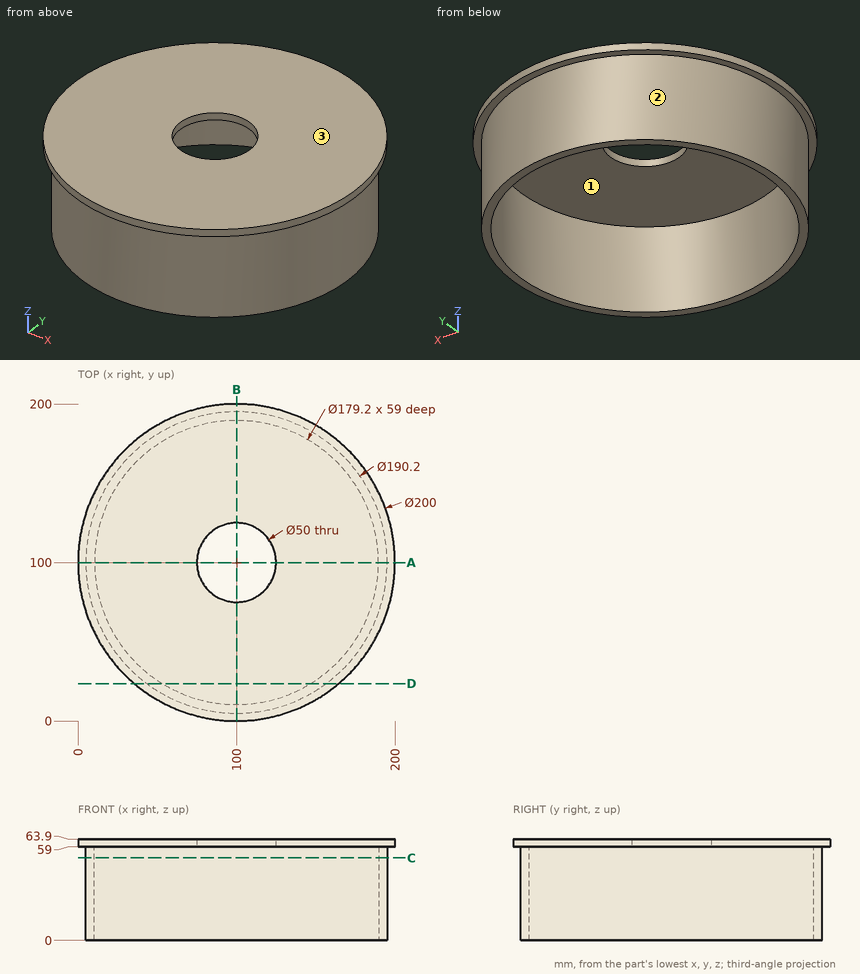
The figure shows three views and two pictorial views of one solid part (mm, origin at its lowest corner). Answer the questions. Give positions to 0.01 mm unless a question says otherwise; leave off trailing zeros. Loops run counter-clockwise (first coordinate to the right, second up) from the corner with the lowest first, then second, coordinate; pieces in that order, holes last. Notation, with made-up numbers: (-5, 73) -> (15, 73) arc R7 cw to (15, 83) -> close; hole circle Ø3 at (77, -6). An arc over 180 degrees is marked (long way). Use CSV: the item, a comma, the result in double quotes.
1. Straight lines are drawn through the part: line 1 (Y direction, x = 100, z = 62); line 2 (Y direction, x = 100, z = 19); line 3 (X direction, y = 120, z = 10.5). For each, find the intervals that lie inside material, in ascending order.
Found:
line 1,"0 to 75, 125 to 200"
line 2,"4.9 to 10.4, 189.6 to 195.1"
line 3,"7.03 to 12.66, 187.34 to 192.97"
2. Flat-ended cylindrical pins translate along their axes: pin 1 Ø8 at (y, z) = (133, 27.5) entering from +X; pin 2 Ø4 at (x, z) = (48.5, 51) entering from +Y; pin 3 Ø5 at (x, z) = (78, 12) entering from -Y. Find the tip coordinate at first contact, or state that the pin passes through.
Found:
pin 1,"x = 190.57"
pin 2,"y = 181.2"
pin 3,"y = 6.92"
3. The part is cut by section D-D (y = 23.5). Write down the section's boundary in (x, z).
Found:
outline,"(35.6, 59) -> (43.5, 59) -> (43.5, 0) -> (53.35, 0) -> (53.35, 59) -> (146.65, 59) -> (146.65, 0) -> (156.5, 0) -> (156.5, 59) -> (164.4, 59) -> (164.4, 63.9) -> (35.6, 63.9) -> close"
4. The part is cut by section C-C (z = 52). Write down the section's boundary in (x, y).
Found:
outline,"circle Ø190.2 at (100, 100); hole circle Ø179.2 at (100, 100)"
5. The part is cut by section A-A (y = 100). Write down the section's boundary in (x, z), then the cut area to 3 significant figures.
Found:
outline,"(0, 59) -> (4.9, 59) -> (4.9, 0) -> (10.4, 0) -> (10.4, 59) -> (75, 59) -> (75, 63.9) -> (0, 63.9) -> close; (125, 59) -> (189.6, 59) -> (189.6, 0) -> (195.1, 0) -> (195.1, 59) -> (200, 59) -> (200, 63.9) -> (125, 63.9) -> close"
area,"1,380 mm^2"
6. The mould has two halves that part along X. Classify the marked faces 1, 2 and 3: +X half, -X half, draft (parallel to the pull), parting line (faces both ways), or undercut.
Found:
face 1,"undercut"
face 2,"parting line"
face 3,"draft"
